Could you check a few things on this drawing? It's one solid part, dimensions in mm from its lowest x, y, z. A direction names the side the tool comes from. Give positions to 0.01 mm unless a question says otherwise; leave off trailing zeros. Write each loop counter-clockwise with the first axis right and the second up, starting at its lowest first coordinate (ties: lowest second). Pieces come first, ordered by that corner, then holes.
1. I'm going to push a flat-ended pin straight in: pin 1 (16.5 mm diameter, centred on y = 96.52, z = 35.56, fed in from +X). Where does the tip first touch, or does it pass through?
2. Suppose I cut it at D-D (x = 60). Please give me the cut outline in (y, z).
3. Suppose I cut it at B-B (z = 25.5). Please give me the cut outline in (x, y).
4. Thinking about a two-plate mould opening in X: for the marked faces 1, 2 and 3, which applies, pulls with the +X half, pulls with the -X half, needs draft (parallel to the pull), parting line crosses it, or undercut?
5. Suppose I cut it at C-C (z = 39). Please give me the cut outline in (x, y), and give its area (3 significant figures).
6. If I drill on probe 1 along X at (y, z) = (93, 64.5); probe 2 along Z at (x, y) = (83, 96); probe 3 along Y at (x, z) = (23, 11), over which ranges is the centre line in solid material (lowest first)?
7. Suppose I cut it at A-A (y = 16). Please give me the cut outline in (x, z), and give its area (3 significant figures).
8. On a 3-axis mill with a long thin cutter (end or side, diameter ignored), from which of +Z, -Z, +X, -X, +Y, -Y can I reach the whole of each face in a straight line? I mean the marked faces 4 and 5. Say none if no direction works.
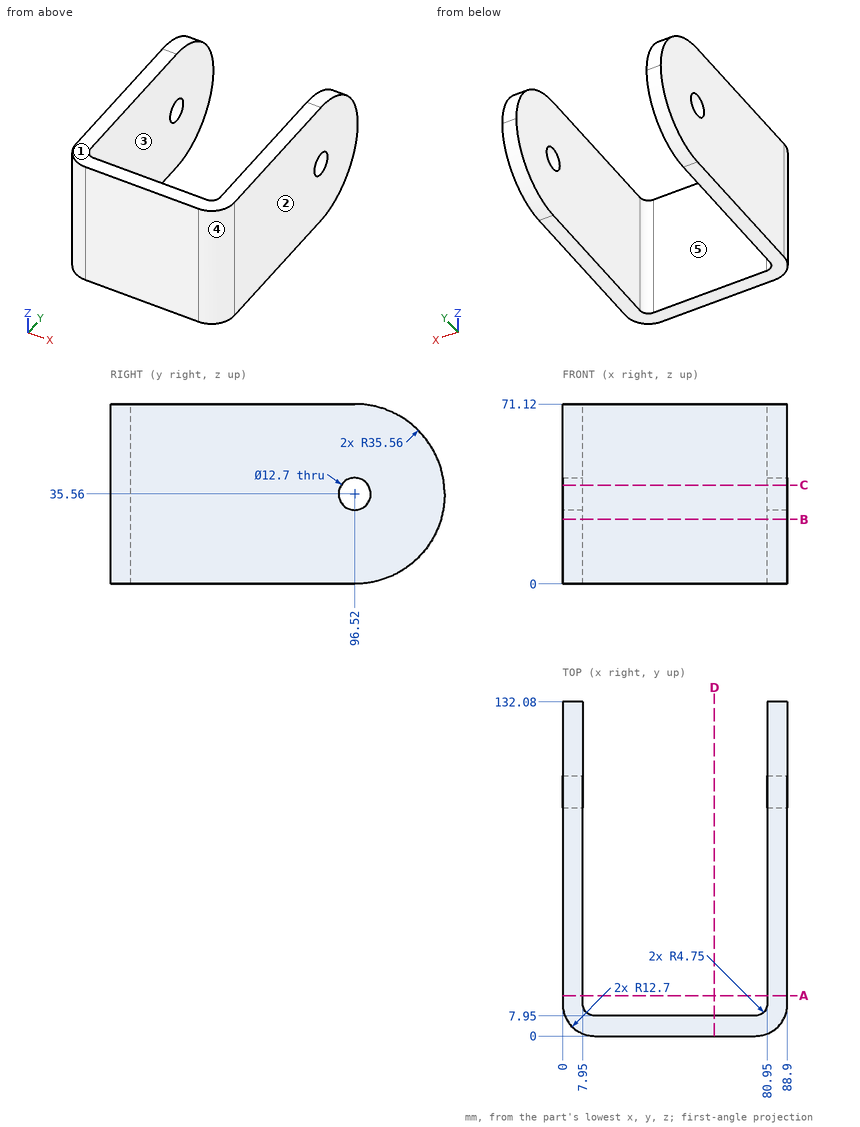
Checks:
1. pin 1: stops at x = 88.9
2. outline: (0, 0) - (7.95, 0) - (7.95, 71.12) - (0, 71.12) - close
3. outline: (0, 12.7) arc R12.7 ccw to (12.7, 0) - (76.2, 0) arc R12.7 ccw to (88.9, 12.7) - (88.9, 130.63) - (80.95, 130.63) - (80.95, 12.7) arc R4.75 cw to (76.2, 7.95) - (12.7, 7.95) arc R4.75 cw to (7.95, 12.7) - (7.95, 130.63) - (0, 130.63) - close
4. face 1: needs draft
4. face 2: pulls with the +X half
4. face 3: undercut
5. outline: (0, 12.7) arc R12.7 ccw to (12.7, 0) - (76.2, 0) arc R12.7 ccw to (88.9, 12.7) - (88.9, 91.18) - (80.95, 91.18) - (80.95, 12.7) arc R4.75 cw to (76.2, 7.95) - (12.7, 7.95) arc R4.75 cw to (7.95, 12.7) - (7.95, 91.18) - (0, 91.18) - close; (0, 101.86) - (7.95, 101.86) - (7.95, 131.91) - (0, 131.91) - close; (80.95, 101.86) - (88.9, 101.86) - (88.9, 131.91) - (80.95, 131.91) - close
5. area: 2,450 mm2
6. probe 1: x = 0 to 7.95, 80.95 to 88.9
6. probe 2: z = 0 to 29.23, 41.89 to 71.12
6. probe 3: y = 0 to 7.95
7. outline: (0, 0) - (7.95, 0) - (7.95, 71.12) - (0, 71.12) - close; (80.95, 0) - (88.9, 0) - (88.9, 71.12) - (80.95, 71.12) - close
7. area: 1,130 mm2
8. face 4: +Z, -Z, +X, -Y
8. face 5: +Z, -Z, +Y
